Autodesk Inventor part; units mm, degrees
ref_plane "YZ Plane" through (0, 0, 0) normal (1, 0, 0) x (0, 1, 0)
ref_plane "XZ Plane" through (0, 0, 0) normal (0, 1, 0) x (-1, 0, 0)
ref_plane "XY Plane" through (0, 0, 0) normal (0, 0, 1) x (1, 0, 0)
sketch "Sketch2" plane through (0, 0, 0) normal (0, 0, 1) x (1, 0, 0)
  line L0 (-32.5, -3.1) -> (-25.5, -3.1)
  line L1 (-25.5, -3.1) -> (-25.5, -7)
  line L2 (-25.5, -7) -> (-32.5, -7)
  line L3 (-32.5, -7) -> (-32.5, -3.1)
  line L4 (-31.2, 0) -> (-26.8, 0)
  line L5 (-26.8, 0) -> (-26.8, -3.1)
  line L6 (-26.8, -3.1) -> (-31.2, -3.1)
  line L7 (-31.2, -3.1) -> (-31.2, 0)
  line L8 (-35.5, 0) -> (0, 0)
  line L9 (0, 5) -> (-35.5, 5)
  line L10 (-35.5, 5) -> (-35.5, 0)
  line L11 (-29, 6.5254) -> (-29, -10.3092) construction
  line L12 (0, -40.9051) -> (0, 14.4305) construction
  line L13 (32.5, -3.1) -> (25.5, -3.1)
  line L14 (25.5, -3.1) -> (25.5, -7)
  line L15 (25.5, -7) -> (32.5, -7)
  line L16 (32.5, -7) -> (32.5, -3.1)
  line L17 (31.2, 0) -> (26.8, 0)
  line L18 (26.8, 0) -> (26.8, -3.1)
  line L19 (26.8, -3.1) -> (31.2, -3.1)
  line L20 (31.2, -3.1) -> (31.2, 0)
  line L21 (35.5, 0) -> (0, 0)
  line L22 (0, 5) -> (35.5, 5)
  line L23 (35.5, 5) -> (35.5, 0)
  line L24 (29, 6.5254) -> (29, -10.3092) construction
  line L25 (-84.7245, 0) -> (105.0676, 0) construction
  line L26 (35.5, 5) -> (77.9544, -30.0249)
  line L27 (77.9544, -30.0249) -> (75.5, -33)
  line L28 (75.5, -33) -> (35.5, 0)
  line L29 (-35.5, 5) -> (35.5, 5)
  line L30 (35.5, 5) -> (35.5, -7)
  line L31 (35.5, -7) -> (-35.5, -7)
  line L32 (-35.5, -7) -> (-35.5, 5)
  line L33 (-35.5, 5) -> (-57.6113, -7.1612)
  line L34 (-57.6113, -7.1612) -> (-55.5, -11)
  line L35 (-55.5, -11) -> (-35.5, 0)
  line L36 (-21.5, -7) -> (-21.5, -4)
  line L37 (-21.5, -4) -> (0, -4)
  line L38 (21.5, -7) -> (21.5, -4)
  line L39 (21.5, -4) -> (0, -4)
  line L40 (-35.5, -7) -> (-48.2273, -7)
  line L41 (35.5, -7) -> (43.9848, -7)
  point P0 (-13.25, 5)
  point P1 (-18.25, 5)
  point P2 (29, -7)
  point P3 (32.5, -7)
  point P4 (-32.5, -7)
  point P5 (21.5, -7)
  dimension "d1" = 4.4
  dimension "d2" = 7
  dimension "d3" = 3.9
  dimension "d4" = 5
  dimension "d5" = 58
  dimension "d6" = 7
  dimension "d7" = 13
  dimension "d28" = 38
  dimension "d29" = 40
  dimension "d30" = 20
  dimension "d31" = 16
  dimension "d37" = 4
  dimension "d38" = 3
extrude "Extrusion1" add sketch "Sketch2" along normal blind 12 contours L0 L1 L2 L3 | L7 L4 L5 L0 | L8 L10 L9 L22 L23 L21 L17 L4 | L35 L34 L33 L10 | L17 L20 L13 L18 | L14 L13 L16 L15 | L26 L27 L28 L23
extrude "Extrusion3" add sketch "Sketch2" against normal blind 3 contours L3 L31 L32 L8 L7 L0 | L0 L1 L2 L3 | L7 L4 L5 L0 | L5 L8 L21 L18 L13 L14 L31 L38 L39 L37 L36 L1 L0 | L8 L10 L9 L22 L23 L21 L17 L4 | L40 L35 L32 | L35 L34 L33 L10 | L17 L20 L13 L18 | L14 L13 L16 L15 | L21 L30 L31 L16 L13 L20 | L26 L27 L28 L23 | L28 L41 L30
sketch "Sketch3" plane through (-57.6113, -7.1612, 12) normal (-0.4819, 0.8762, 0) x (0.8762, 0.4819, 0)
  circle A0 centre (8, 7.5) radius 2
  line L0 (0, 0) -> (0, 15)
  line L1 (25.235, 0) -> (0, 0)
  point P0 (53.9311, 12)
  dimension "d39" = 4
  dimension "d40" = 8
  dimension "d41" = 7.5
extrude "Extrusion4" cut sketch "Sketch3" against normal blind 10
sketch "Sketch4" plane through (35.5, 5, 12) normal (0.6364, 0.7714, 0) x (0.7714, -0.6364, 0)
  circle A0 centre (47.0375, 7.5) radius 2
  line L0 (55.0375, 15) -> (55.0375, 0)
  line L1 (0, 15) -> (55.0375, 15)
  point P0 (-24.2018, 12)
  dimension "d44" = 4
  dimension "d45" = 8
  dimension "d46" = 7.5
extrude "Extrusion5" cut sketch "Sketch4" against normal blind 10
properties part number "UnitreeGO2_railmount"
Geometry check sheet. Reference: the model listing, model coordinates, mm. A direction names the side the tool comes from. Round coordinates to 2 decimals unless told otherwise and drop trailing zeros. Loops run counter-clockwise (first coordinate to the right, second up) from the corner with the lowest first, then second, coordinate; pieces in that order, holes last.
Item 1: Access from +Z, -Z, +X, -X, +Y, -Y to the whole of each face (thin tool, end or side, straight path). Record for faces 5 (the flat face through (30, -7, 1)), 6 (the flat face through (5, -3, -3)), 7 (the flat face through (26.8, -2, 6)), 8 (the flat face through (32.5, -5, 6)).
Item 2: Thickness scan on line 1 (Y direction, x = -31.5, z = 10); line 2 (X direction, y = -6.5, z = 4.5); line 3 (X direction, y = -5, z = 2). Record the ranges inside material, lowest first.
Item 3: Gauge pin test, flat ends, axial feed: pin 1 (1.5 mm diameter, centred on x = -30, z = -0.5, fed in from -Y); pin 2 (1.5 mm diameter, centred on y = -1.5, z = -1, fed in from -X); pin 3 (1.5 mm diameter, centred on x = 10.5, z = -1, fed in from -Y). Record the tip position at first contact, or that the pin passes through.
Item 4: Cross-section at C-C on y = -17.5. Record the boundary of the cut face in (x, z).
Item 5: Cross-section at D-D on x = -38. Record the boundary of the cut face in (y, z) (3 decimals).
Item 6: Cross-section at A-A on x = -2.5. Record the boundary of the cut face in (y, z).
Item 7: Mould release check, pull along X, two halves, no side actions. Record for faces 1 (the cylindrical face through (71.29, -26.99, 6.27)), 2 (the flat face through (56.43, -12.267, 4.395)), 3 (the flat face through (-56.57, -9.054, 4.395)), 4 (the flat face through (-33, 0, 6)): pulls with the +X half, pulls with the -X half, needs draft (parallel to the pull), parting line crosses it, or undercut.
Item 8: Cross-section at B-B on z = 10. Record the boundary of the cut face in (x, y).
Answer sheet:
1. face 5: +Z, -Z, -Y
1. face 6: -Z, +X, -X, +Y, -Y
1. face 7: +Z
1. face 8: +Z, -Y
2. line 1: y = -7 to -3.1, 0 to 5
2. line 2: x = -56.41 to -51.13, -32.5 to -25.5, 25.5 to 32.5, 43.38 to 49.44
2. line 3: x = -53.68 to -44.59, -32.5 to -25.5, 25.5 to 32.5, 41.56 to 47.62
3. pin 1: stops at y = -7
3. pin 2: stops at x = -48.68
3. pin 3: stops at y = -4
4. outline: (56.71, -3) - (62.77, -3) - (62.77, 12) - (56.71, 12) - close
5. outline: (-7, -3) - (3.625, -3) - (3.625, 12) - (-1.375, 12) - (-1.375, 0) - (-7, 0) - close
6. outline: (-4, -3) - (5, -3) - (5, 12) - (0, 12) - (0, 0) - (-4, 0) - close
7. face 1: undercut
7. face 2: pulls with the +X half
7. face 3: pulls with the -X half
7. face 4: undercut
8. outline: (-57.61, -7.16) - (-55.5, -11) - (-35.5, 0) - (-31.2, 0) - (-31.2, -3.1) - (-32.5, -3.1) - (-32.5, -7) - (-25.5, -7) - (-25.5, -3.1) - (-26.8, -3.1) - (-26.8, 0) - (26.8, 0) - (26.8, -3.1) - (25.5, -3.1) - (25.5, -7) - (32.5, -7) - (32.5, -3.1) - (31.2, -3.1) - (31.2, 0) - (35.5, 0) - (75.5, -33) - (77.95, -30.02) - (35.5, 5) - (-35.5, 5) - close
